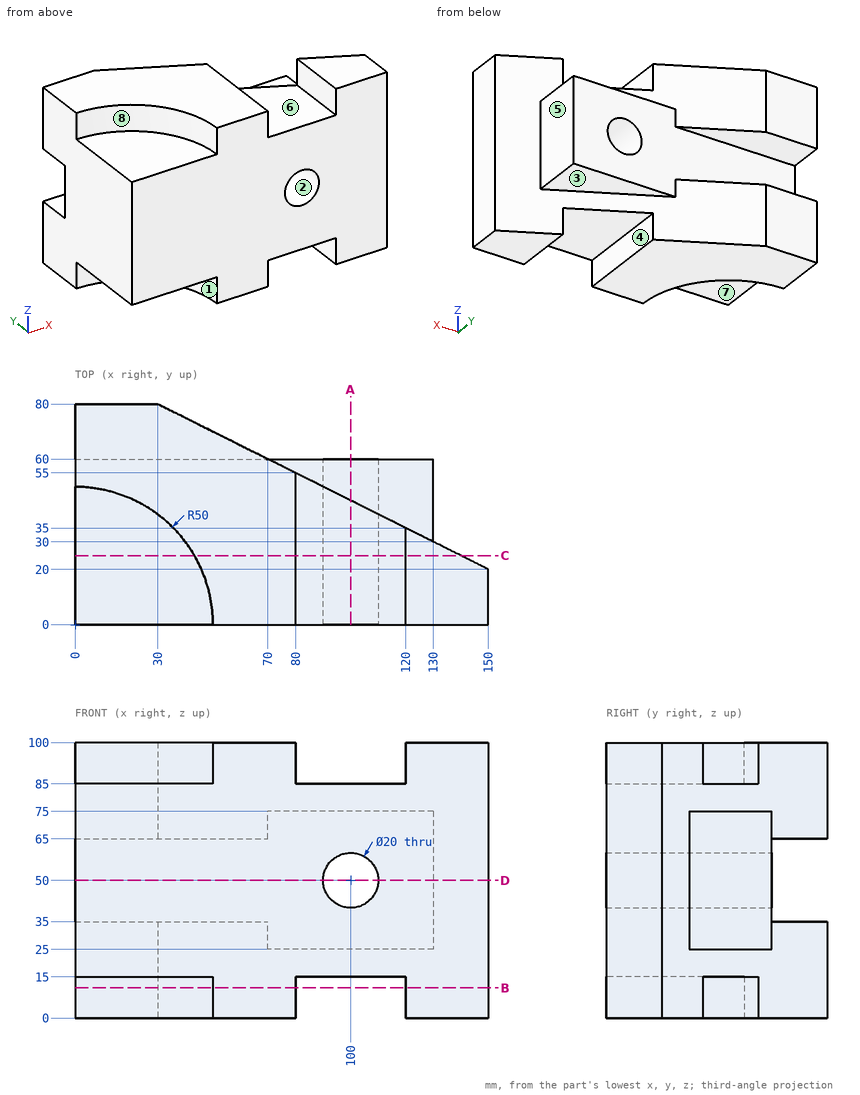
Geometry: see drawing. Coordinates: mm, zero at the bounding-box minimum. A direction names the side the tool comes from. Round coordinates to 2 decimals unless told otherwise and drop trailing zeros. Loops run counter-clockwise (first coordinate to the right, second up) from the corner with the lowest first, then second, coordinate; pieces in that order, holes last. Notation, with made-up numbers: (42, 87.5) -> (52, 87.5) arc R24 ccw to (52, 111.5) -> close; hole circle Ø5 at (-23, -5). An arc over 180 degrees is marked (long way). One line per question, with ' | ' between items. Start each with the question number.
1. Mould query, pull axis Z, two halves, no side actions, for the marked faces 1, 2 and 3. Classes: pulls with the +Z half, pulls with the -Z half, needs draft (parallel to the pull), parting line crosses it, or undercut.
2. Section B-B on z = 11. Output: boundary loops of the cut face in (x, y).
3. Set-up query: the marked faces 4, 5, 6, 7 and 8. Return all of +Z, -Z, +X, -X, +Y, -Y with unobstructed straight access to the full face (end or side cutting, diameter ignored); none if empty.
4. Contact query for flat-ended pins moving along their axis: pin 1 (12 mm diameter, centred on x = 25.5, z = 55, fed in from +Y); pin 2 (15 mm diameter, centred on y = 45.5, z = 45.5, fed in from +X); pin 3 (7.5 mm diameter, centred on y = 19.5, z = 91.5, fed in from -X). Output: stop coordinate, or through.
5. Section C-C on y = 25. Output: boundary loops of the cut face in (x, z).
6. Section A-A on x = 100. Output: boundary loops of the cut face in (y, z).
7. Section D-D on z = 50. Output: boundary loops of the cut face in (x, y).
8. Line query: line 1 along Z through (x, y) = (100, 38.5); line 2 along X through (y, z) = (40, 50); line 3 along Z through (x, y) = (26.5, 63.5). Output: solid intervals per line, ascending. Write a range as [from, to].
Returned:
1) face 1: needs draft | face 2: undercut | face 3: pulls with the -Z half
2) outline: (0, 50) arc R50 cw to (50, 0) -> (80, 0) -> (80, 55) -> (30, 80) -> (0, 80) -> close; (120, 0) -> (150, 0) -> (150, 20) -> (120, 35) -> close
3) face 4: -Z, +Y, -Y | face 5: +Z, -Z, +X, +Y | face 6: +Z, +Y, -Y | face 7: -Z, -X, -Y | face 8: +Z, -X, -Y
4) pin 1: stops at y = 60 | pin 2: stops at x = 130 | pin 3: stops at x = 44.27
5) outline: (0, 15) -> (43.3, 15) -> (43.3, 0) -> (80, 0) -> (80, 15) -> (120, 15) -> (120, 0) -> (140, 0) -> (140, 100) -> (120, 100) -> (120, 85) -> (80, 85) -> (80, 100) -> (43.3, 100) -> (43.3, 85) -> (0, 85) -> close; hole circle Ø20 at (100, 50)
6) outline: (0, 15) -> (45, 15) -> (45, 25) -> (60, 25) -> (60, 40) -> (0, 40) -> close; (0, 60) -> (60, 60) -> (60, 75) -> (45, 75) -> (45, 85) -> (0, 85) -> close
7) outline: (0, 0) -> (90, 0) -> (90, 60) -> (0, 60) -> close; (110, 0) -> (150, 0) -> (150, 20) -> (130, 30) -> (130, 60) -> (110, 60) -> close
8) line 1: z = [15, 40], [60, 85] | line 2: x = [0, 90], [110, 130] | line 3: z = [0, 35], [65, 100]
